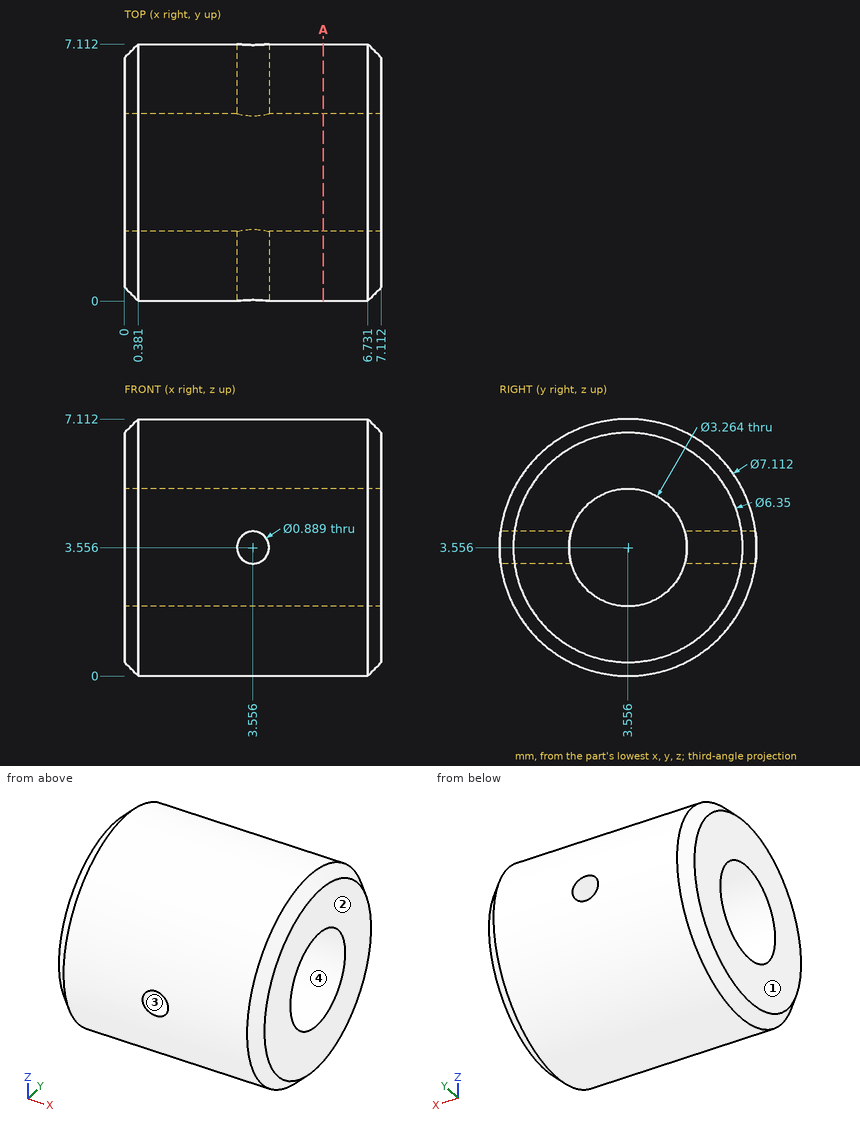
Input: dimensioned drawing with shaded views. Units: mm. Origin: part minimum x, y, z. Give positions to 0.01 mm unless a question says otherwise; leave off trailing zeros. Loops run counter-clockwise (first coordinate to the right, second up) from the corner with the lowest first, then second, coordinate; pieces in that order, holes last. Notation, with made-up numbers: M 57,-4.5 L 94,-4.5 A23 cw 94,8.5 Z; hole C 31,-11 d10. An arc over 180 degrees is marked long. Put each result on its own line as item: value. Start each with the question number.
1) Cut plane A-A (x = 5.5). Output: boundary loops of the cut face in (y, z), then the cut area to 3 significant figures.
2) Pull-direction query (X, two-part tool) for the marked faces 1, 2, 3 and 4; classes: pulls with the +X half, pulls with the -X half, needs draft (parallel to the pull), parting line crosses it, or undercut.
3) Ray query, line 1 along Z through (x, y) = (2.25, 4); line 2 along Y through (x, z) = (5, 5) (1 decimal); line 3 along Y through (x, z) = (2.75, 3). Return the intervals inside material, ascending.
Verdict:
1. outline: C 3.56,3.56 d7.11; hole C 3.56,3.56 d3.26
1. area: 31.4 mm2
2. face 1: pulls with the -X half
2. face 2: pulls with the +X half
2. face 3: undercut
2. face 4: needs draft
3. line 1: 0.03 to 1.99, 5.13 to 7.08
3. line 2: 0.3 to 2.8, 4.3 to 6.8
3. line 3: 0.04 to 2.02, 5.09 to 7.07
